Autodesk Inventor part; units mm, degrees
ref_plane "YZ Plane" through (0, 0, 0) normal (1, 0, 0) x (0, 1, 0)
ref_plane "XZ Plane" through (0, 0, 0) normal (0, 1, 0) x (-1, 0, 0)
ref_plane "XY Plane" through (0, 0, 0) normal (0, 0, 1) x (1, 0, 0)
sketch "Sketch1" plane through (0, 0, 0) normal (1, 0, 0) x (0, 1, 0)
  line L0 (-14.5, 15) -> (-14.5, -15)
  line L1 (-14.5, -15) -> (14.5, -15)
  arc A0 (14.5, -15) -> (14.5, 15) centre (14.5, 0) ccw
  line L2 (14.5, 15) -> (-14.5, 15)
  circle A1 centre (14.5, 0) radius 5
  point P0 (0, 0)
  point P1 (0, -15)
  dimension "d0" = 15
  dimension "d1" = 10
  dimension "d2" = 29
extrude "Extrusion1" add sketch "Sketch1" along normal mid plane 40
sketch "Sketch2" plane through (0, 0, 0) normal (0, 0, 1) x (1, 0, 0)
  line L0 (-20, 14.5) -> (20, 14.5) construction
  line L1 (20, 14.5) -> (20, 14.5) construction
  line L2 (-20, 14.5) -> (20, 14.5) construction
  line L3 (-20, 14.5) -> (-20, 14.5) construction
  line L4 (-20, 14.5) -> (20, 14.5) construction
  line L5 (20, -14.5) -> (20, 14.5) construction
  line L6 (20, -14.5) -> (-20, -14.5) construction
  line L7 (-20, 14.5) -> (-20, -14.5) construction
  line L8 (-10, 29.5) -> (10, 29.5)
  line L9 (10, 29.5) -> (10, -4.5)
  line L10 (10, -4.5) -> (-10, -4.5)
  line L11 (-10, -4.5) -> (-10, 29.5)
  line L12 (-20, 29.5) -> (20, 29.5) construction
  point P0 (0, 0)
  point P1 (0, 29.5)
  dimension "d5" = 20
  dimension "d6" = 10
  dimension "d7" = 34
extrude "Extrusion2" cut sketch "Sketch2" along normal mid plane 40
sketch "Sketch3" plane through (0, 0, 0) normal (0, 1, 0) x (-1, 0, 0)
  circle A0 centre (0, 0) radius 4.3
  dimension "d10" = 8.6
extrude "Extrusion3" cut sketch "Sketch3" against normal through all
properties part number "cuerpo_obj3"
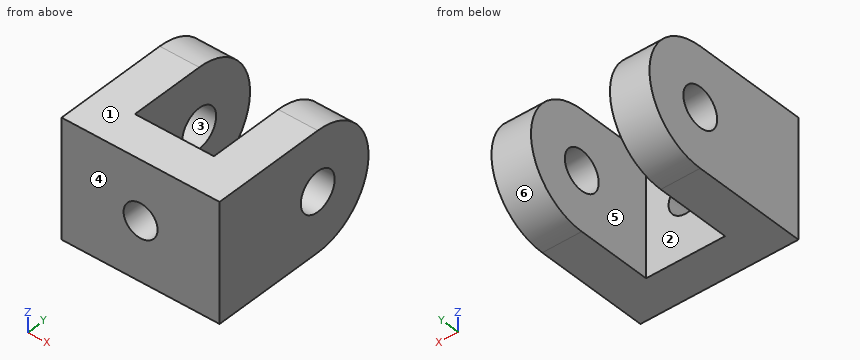
Input: part model. Units: mm. Frame: model coordinates. Face numbers are marked on the shaded views. A direction names the side the tool comes from. Give positions to 0.01 mm unless a question says otherwise; leave off trailing zeros. Write each loop counter-clockwise with the first axis right and the second up, starting at its lowest first coordinate (ties: lowest second). Pieces come first, ordered by that corner, then holes. Notation, with made-up numbers: M -15,12.25 L 25,12.25 A23 ccw 25,45.25 Z; hole C 17,-31 d10. An arc over 180 degrees is marked long. Use one line per item in the form item = value.
1. Cut plane A-A on x = 0. Return loops of the section in (y, z), and give its area (3 significant figures).
Outcome:
outline = M -14.5,-15 L -4.5,-15 L -4.5,-4.3 L -14.5,-4.3 Z; M -14.5,4.3 L -4.5,4.3 L -4.5,15 L -14.5,15 Z
area = 214 mm²
2. Cut plane D-D on y = 12. Return loops of the section in (x, z).
Outcome:
outline = M -20,-15 L -10,-15 L -10,-4.33 L -20,-4.33 Z; M -20,4.33 L -10,4.33 L -10,15 L -20,15 Z; M 10,-15 L 20,-15 L 20,-4.33 L 10,-4.33 Z; M 10,4.33 L 20,4.33 L 20,15 L 10,15 Z
3. Mould query, pull axis Y, two halves, no side actions, for the marked faces 3, 4, 5 and 6. Classes: released by +Y, released by -Y, zero draft, split by the parting line, or undercut.
Outcome:
face_3 = undercut
face_4 = released by -Y
face_5 = zero draft
face_6 = released by +Y
4. Ray query, L1, parallel to Z at x = -12.25, y = 14.5; L2, parallel to Y at x = -13.5, z = 0; L3, parallel to X at y = 7.5, z = -5.75. Return the intervals inside material, ascending.
Outcome:
L1 = -15 to -5, 5 to 15
L2 = -14.5 to 9.5, 19.5 to 29.5
L3 = -20 to -10, 10 to 20
5. First-contact query: P1, Ø3, axis at x = -11, z = 8.5, coming from the +Y side; P2, Ø2, axis at x = 7.5, y = 13.5, coming from the -Z side; P3, Ø1.5, axis at x = 7, z = -11.5, coming from the +Y side; P4, Ø15, axis at y = 14.5, z = -4, coming from the -X side. Flat tips, straight axial feed; report the tip coordinate or a pass-through.
Outcome:
P1 = 27.77
P2 = through
P3 = -4.5
P4 = -20
6. Cut plane C-C on z = 0. Return loops of the section in (x, y), and give its area (3 significant figures).
Outcome:
outline = M -20,-14.5 L -4.3,-14.5 L -4.3,-4.5 L -10,-4.5 L -10,9.5 L -20,9.5 Z; M -20,19.5 L -10,19.5 L -10,29.5 L -20,29.5 Z; M 4.3,-14.5 L 20,-14.5 L 20,9.5 L 10,9.5 L 10,-4.5 L 4.3,-4.5 Z; M 10,19.5 L 20,19.5 L 20,29.5 L 10,29.5 Z
area = 794 mm²
7. Cut plane B-B on y = 1.5. Return loops of the section in (x, z).
Outcome:
outline = M -20,-15 L -10,-15 L -10,15 L -20,15 Z; M 10,-15 L 20,-15 L 20,15 L 10,15 Z
8. Reachability of the marked faces 1 and 2 from +Z, -Z, +X, -X, +Y, -Y: full face, straight path, thin tool, end or side. Return the list, or none.
Outcome:
face_1 = +Z, +X, -X, +Y, -Y
face_2 = +Z, -Z, +Y
